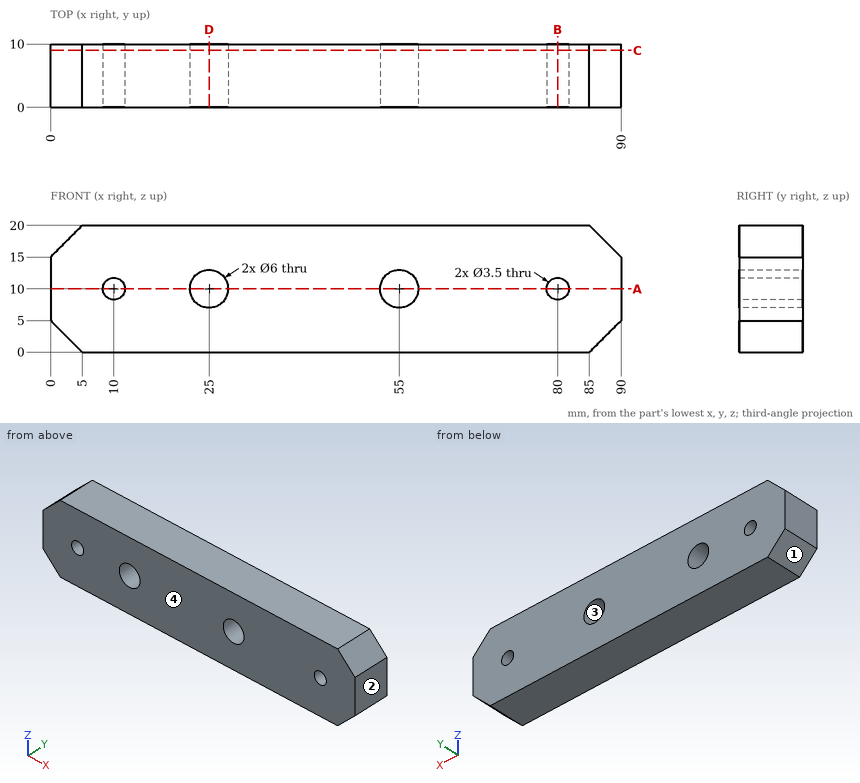
Job drawing, mm, ordinate dimensions from the low corner. One solid piece. Give positions to 0.01 mm unless a question says otherwise; leave off trailing zeros. Loops run counter-clockwise (first coordinate to the right, second up) from the corner with the lowest first, then second, coordinate; pieces in that order, holes last. Notation, with made-up numbers: (4.25, 62) -> (33.25, 62) arc R14 ccw to (33.25, 85) -> close; hole circle Ø2 at (12.5, -17). An arc over 180 degrees is marked (long way). Use a Markdown table: item, result. Add a question column.
(1) Slice it at C-C on y = 9. List the corners of the cut face in (x, z), and give its area (3 significant figures).
(2) Drop a flat-ended pin along its axis: pin 1 Ø2 at (x, z) = (10, 10) entering from +Y. Give the stop position or say it passes through.
(3) Slice it at B-B on x = 80. List the corners of the cut face in (y, z).
(4) Wall check: line 1 along X through (y, z) = (6, 10); line 2 along X through (y, z) = (7.5, 8); line 3 along X through (y, z) = (1, 8.5). Give the ranges that are in metal, low to high.
(5) Slice it at A-A on z = 10. List the corners of the cut face in (x, y).
(6) Mould opens along X. For the marked faces 1, 2, 3 and 4 say: +X half, -X half, draft (parallel to the pull), parting line (faces both ways), or undercut.
(7) Slice it at D-D on x = 25. List the corners of the cut face in (y, z), and give its area (3 significant figures).
Filled sheet:
| question | item | result |
|---|---|---|
| 1 | outline | (0, 5) -> (5, 0) -> (85, 0) -> (90, 5) -> (90, 15) -> (85, 20) -> (5, 20) -> (0, 15) -> close; hole circle Ø3.5 at (10, 10); hole circle Ø6 at (25, 10); hole circle Ø6 at (55, 10); hole circle Ø3.5 at (80, 10) |
| 1 | area | 1,670 mm2 |
| 2 | pin 1 | through |
| 3 | outline | (0, 0) -> (10, 0) -> (10, 8.25) -> (0, 8.25) -> close; (0, 11.75) -> (10, 11.75) -> (10, 20) -> (0, 20) -> close |
| 4 | line 1 | 0 to 8.25, 11.75 to 22, 28 to 52, 58 to 78.25, 81.75 to 90 |
| 4 | line 2 | 0 to 22.76, 27.24 to 52.76, 57.24 to 90 |
| 4 | line 3 | 0 to 9.1, 10.9 to 22.4, 27.6 to 52.4, 57.6 to 79.1, 80.9 to 90 |
| 5 | outline | (0, 0) -> (8.25, 0) -> (8.25, 10) -> (0, 10) -> close; (11.75, 0) -> (22, 0) -> (22, 10) -> (11.75, 10) -> close; (28, 0) -> (52, 0) -> (52, 10) -> (28, 10) -> close; (58, 0) -> (78.25, 0) -> (78.25, 10) -> (58, 10) -> close; (81.75, 0) -> (90, 0) -> (90, 10) -> (81.75, 10) -> close |
| 6 | face 1 | -X half |
| 6 | face 2 | +X half |
| 6 | face 3 | undercut |
| 6 | face 4 | draft |
| 7 | outline | (0, 0) -> (10, 0) -> (10, 7) -> (0, 7) -> close; (0, 13) -> (10, 13) -> (10, 20) -> (0, 20) -> close |
| 7 | area | 140 mm2 |
